```python
from build123d import *

# Parameters (mm, degrees)
SKETCH_1_W               = 4.5
SKETCH_1_H               = 3.99
EXTRUDE_1_DEPTH          = 6
SKETCH_1_3_W             = 4.5
SKETCH_1_3_H             = 3.99
CUT_EXTRUDE_1_DEPTH      = 1
HOLE_WIZARD_M2_10_D      = 1.6
CUT_EXTRUDE_2_DEPTH      = 98.948437456
CUT_EXTRUDE_2_DEPTH_BACK = 98.948437456
SKETCH_19_W              = 3.2
SKETCH_19_H              = 3.5
FILLET_2_R               = 0.5


with BuildPart() as part:
    # Sketch 1 → Extrude 1 (new body)
    with BuildSketch(Plane.XY):
        with Locations((72.17, 48.655)):
            Rectangle(SKETCH_1_W, SKETCH_1_H)
        Polygon((74.42, 50.65), (74.42, 63.4), (0, 63.4), (0, 0), (74.42, 0), (74.42, 46.66), (69.92, 46.66), (69.92, 50.65), align=None)
    extrude(amount=-EXTRUDE_1_DEPTH)

    # Sketch 1_3 → Cut-Extrude 1 (cut)
    with BuildSketch(Plane.XY):
        with Locations((72.17, 48.655)):
            Rectangle(SKETCH_1_3_W, SKETCH_1_3_H)
    extrude(amount=-CUT_EXTRUDE_1_DEPTH, mode=Mode.SUBTRACT)

    # Hole Wizard M2 _10 (through all)
    with Locations(Plane.XY):
        with Locations((3.61, 61.113), (72.488, 61.113), (72.488, 2.851), (3.61, 2.851)):
            Hole(HOLE_WIZARD_M2_10_D / 2)

    # Sketch 19 → Cut-Extrude 2 (cut, two sides: drawn at the far end of the back side and taken through both)
    with BuildSketch(Plane.XZ.offset(-CUT_EXTRUDE_2_DEPTH_BACK)):
        with Locations((9.1, -4.25)):
            Rectangle(SKETCH_19_W, SKETCH_19_H)
        with Locations((15.5, -4.25)):
            Rectangle(SKETCH_19_W, SKETCH_19_H)
        with Locations((21.9, -4.25)):
            Rectangle(SKETCH_19_W, SKETCH_19_H)
        with Locations((28.3, -4.25)):
            Rectangle(SKETCH_19_W, SKETCH_19_H)
        with Locations((34.7, -4.25)):
            Rectangle(SKETCH_19_W, SKETCH_19_H)
        with Locations((41.1, -4.25)):
            Rectangle(SKETCH_19_W, SKETCH_19_H)
        with Locations((47.5, -4.25)):
            Rectangle(SKETCH_19_W, SKETCH_19_H)
        with Locations((53.9, -4.25)):
            Rectangle(SKETCH_19_W, SKETCH_19_H)
        with Locations((60.3, -4.25)):
            Rectangle(SKETCH_19_W, SKETCH_19_H)
        with Locations((66.7, -4.25)):
            Rectangle(SKETCH_19_W, SKETCH_19_H)
    extrude(amount=CUT_EXTRUDE_2_DEPTH + CUT_EXTRUDE_2_DEPTH_BACK, mode=Mode.SUBTRACT)

    # Fillet 2
    fillet_2_edges = [part.edges().sort_by_distance(p)[0] for p in [
        (10.7, 31.7, -6),
        (7.5, 31.7, -6),
        (13.9, 31.7, -6),
        (17.1, 31.7, -6),
        (20.3, 31.7, -6),
        (23.5, 31.7, -6),
        (26.7, 31.7, -6),
        (29.9, 31.7, -6),
        (33.1, 31.7, -6),
        (36.3, 31.7, -6),
        (39.5, 31.7, -6),
        (42.7, 31.7, -6),
        (45.9, 31.7, -6),
        (49.1, 31.7, -6),
        (52.3, 31.7, -6),
        (55.5, 31.7, -6),
        (58.7, 31.7, -6),
        (61.9, 31.7, -6),
        (65.1, 31.7, -6),
        (68.3, 31.7, -6),
    ]]
    fillet(fillet_2_edges, radius=FILLET_2_R)


solid = part.part
```
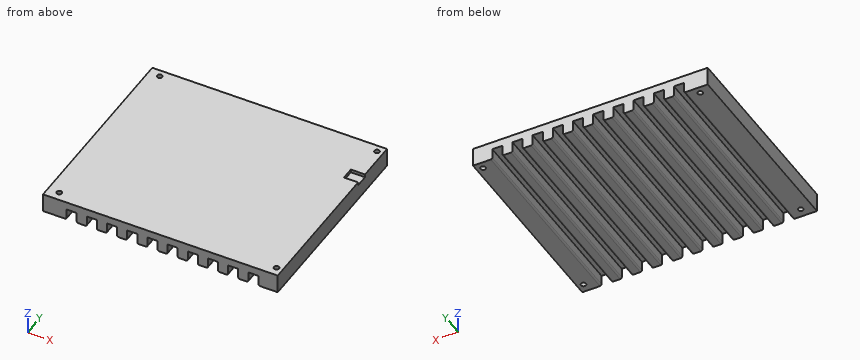
For this review, take the finished solid that the model builds, in its own axes (mm). Give positions to 0.01 mm unless a question says otherwise; leave off trailing zeros. Write each loop counter-clockwise with the first axis right and the second up, starting at its lowest first coordinate (ties: lowest second). Pieces come first, ordered by that corner, then holes. Notation, with made-up numbers: M 4,64.25 L 37,64.25 A26 ccw 37,86.25 Z; hole C 87.25,-12 d6. An arc over 180 degrees is marked long. One line per item, written item: value.
1) Take a section at B-B, the plane x = 28. Write out the cut boundary in (y, z).
Results are:
outline: M 0,-2.5 L 63.4,-2.5 L 63.4,0 L 0,0 Z
2) For line 1 (Y direction, x = 3.61, z = -2.7); line 2 (Z direction, x = 15, y = 24), list the stretches that pass through material, from the lowest coordinate up. Write a range as from..to.
Results are:
line 1: y = 0..2.05, 3.65..60.31, 61.91..63.4
line 2: z = -2.5..0
3) Take a section at A-A, the plane x = 3.61. Write out the cut boundary in (y, z), then the cut area to 3 significant figures.
Results are:
outline: M 0,-6 L 2.05,-6 L 2.05,0 L 0,0 Z; M 3.65,-6 L 60.31,-6 L 60.31,0 L 3.65,0 Z; M 61.91,-6 L 63.4,-6 L 63.4,0 L 61.91,0 Z
area: 361 mm²
4) For P1, Ø1, axis at x = 3.61, y = 61.113, coming from the +Z side; P2, Ø3.5, axis at x = 66.5, y = 21.5, coming from the -Z side, all flat-tipped, find the tip position at first contact; note any pin that passes through.
Results are:
P1: passes through
P2: stops at z = -5.98
